Autodesk Inventor part; units mm, degrees
ref_plane "Work Plane1" through (30.1625, 0, 0) normal (0, 0, -1) x (1, 0, 0)
ref_plane "YZ Plane" through (0, 0, 0) normal (1, 0, 0) x (0, 1, 0)
ref_plane "XZ Plane" through (0, 0, 0) normal (0, 1, 0) x (-1, 0, 0)
sketch "Szkic1" plane through (0, 0, 0) normal (0, 0, 1) x (1, 0, 0)
  line L0 (-6, 0) -> (12, 0)
  line L1 (12, 0) -> (12, 5)
  line L2 (12, 5) -> (3, 5)
  line L3 (3, 5) -> (2.0797, 4.54)
  line L4 (2.0797, 4.54) -> (0, 4.54)
  line L5 (0, 4.54) -> (0, 8)
  line L6 (-9.6, 0) -> (15.6, 0)
  line L7 (0, -1.6) -> (0, 9.6)
  line L8 (-6, 0) -> (-6, 7.4751)
  line L9 (0, 8) -> (-6, 7.4751)
  line L10 (3, 5) -> (0, 5) construction
  dimension "d0" = 12
  dimension "d1" = 9
  dimension "d2" = 0.9203
  dimension "d3" = 6
  dimension "d4" = 10
  dimension "d5" = 9.08
  dimension "d9" = 16
  dimension "d10" = 5
revolve "Bryła" add sketch "Szkic1" angle 360 about axis through (-6, 0, 0) along (1, 0, 0)
sketch "Szkic2" plane through (-6, 0, 0) normal (-1, 0, 0) x (0, 0, 1)
  circle A0 centre (0, 0) radius 8
  line L0 (0, 0) -> (0, 7.4751)
  line L1 (-8, 1.25) -> (8, 1.25)
  line L2 (8, 1.25) -> (8, -1.25)
  line L3 (8, -1.25) -> (-8, -1.25)
  line L4 (-8, -1.25) -> (-8, 1.25)
  line L5 (-8, 0) -> (8, 0) construction
  line L6 (0, 1.25) -> (0, -1.25) construction
  dimension "d11" = 2.5
  dimension "d12" = 16
fillet "Zaokrąglenie1" radius 0.4 1 edges at (-6, -7.4751, 0)
extrude "Szczelina" cut sketch "Szkic2" against normal blind 2.4 contours A0 L3 L1 | L2 L3 A0 | A0 L1 L2 | A0 L4 L1 | L3 L4 A0
thread "Gwint"
chamfer "Faza1" distance 0.9202 distance2 0.9203 1 edges at (12, -5, 0) measured on face at (12, -0.8193, 1.889)
ref_plane "Work Plane1" through (30.1625, 0, 0) normal (0, 0, -1) x (1, 0, 0)
equation "\"d11\" = SBR"
equation "\"d12\" = KOD"
equation "\"d14\" = RR"
equation "\"d19\" = STI"
equation "\"d15\" = GEL"
equation "\"d17\" = -0.5 * SPD + 0.5 * GD"
equation "\"d0\" = NLG"
equation "\"d1\" = GEL"
equation "\"d3\" = KOH"
equation "\"d4\" = GD"
equation "\"d5\" = BDM"
equation "\"d9\" = KOD"
equation "\"d10\" = KEWI"
equation "\"GD\" = NND"
equation "\"NLG\" = 12"
equation "\"GEL\" = 9"
equation "\"KOD\" = 16"
equation "\"KOH\" = 6"
equation "\"GAL\" = 0.61345 * PTC"
equation "\"SPD\" = NND - 1.2269 * PTC"
equation "\"BDM\" = 9.08"
equation "\"GUL\" = 0.61345 * PTC"
equation "\"RR\" = 0.4"
equation "\"SBR\" = 2.5"
equation "\"STI\" = 2.4"
equation "\"KEWI\" = 5deg"
equation "\"PTC\" = 1.5"
equation "\"TOA\" = 30deg"
equation "\"GD1\" = THREADDIA - 1.2269 * PTC"
properties part number "ISO 1207 - M10 x 12" material "Stal nierdzewna 440C"
Read the model definition and answer for the solid it produces. Units are mm, in the model's axes. A direction names the side the tool comes from. Coordinates: 2 decimals unless noted, no trailing zeros. Loops run counter-clockwise (first coordinate to the right, second up) from the corner with the lowest first, then second, coordinate; pieces in that order, holes last. Notation, with made-up numbers: (32, -2.5) -> (41, -2.5) arc R38 cw to (41, 36.5) -> close; hole circle Ø2 at (-6, -18.75). An arc over 180 degrees is marked (long way). Write item = value, one per line. Start each with the question number.
1) The part is cut by section B-B, the plane y = 0. Determine the outline of the cut face in (x, z), plus the area to 3 significant figures.
2) Given P1, Ø3, axis at x = 7.5, z = -6, coming from the +Y side; P2, Ø1.9, axis at x = -5.5, z = 0, coming from the +Y side; P3, Ø3, axis at x = 8.5, z = -6, coming from the -Y side; P4, Ø6, axis at x = -1, z = 0.5, coming from the +Y side, each flat-ended and moving along its own axis, determine where each tip first touches the part or whether it passes through.
3) The part is cut by section A-A, the plane z = 0. Determine the outline of the cut face in (x, y).
4) Find the intervals of material crossed by L1, parallel to Y at x = -4.5, z = -0.5; L2, parallel to Y at x = 8.5, z = 0.25; L3, parallel to X at y = 0, z = -0.25, in increasing order. Write a range as from..to.
5) The mould has two halves that part along Y. Classify faces 4 (the face through (-3.4, -1.67, -7.52)), 5 (the face through (-5, -1.25, 0)), 6 (the face through (12, 0, 0)): pulls with the +Y half, pulls with the -Y half, needs draft (parallel to the pull), parting line crosses it, or undercut.
6) For faces 1 (the face through (1.025, -3.603, 2.763)), 2 (the face through (-3.6, 0, 0)), 3 (the face through (6.98, -1.08, 4.88)), determine the directions among +Z, -Z, +X, -X, +Y, -Y from which every point of the face is accessible in a straight line to the end or side of a thin tool.
7) The part is cut by section C-C, the plane x = 3.75. Determine the outline of the cut face in (y, z).
Result:
q1.outline = (-3.6, -7.69) -> (0, -8) -> (0, -4.54) -> (2.08, -4.54) -> (3, -5) -> (11.08, -5) -> (12, -4.08) -> (12, 4.08) -> (11.08, 5) -> (3, 5) -> (2.08, 4.54) -> (0, 4.54) -> (0, 8) -> (-3.6, 7.69) -> close
q1.area = 173 mm²
q2.P1 = 2.18
q2.P2 = 7.6
q2.P3 = -2.18
q2.P4 = 8
q3.outline = (-6, -7.11) arc R0.4 ccw to (-5.63, -7.51) -> (0, -8) -> (0, -4.54) -> (2.08, -4.54) -> (3, -5) -> (11.08, -5) -> (12, -4.08) -> (12, 4.08) -> (11.08, 5) -> (3, 5) -> (2.08, 4.54) -> (0, 4.54) -> (0, 8) -> (-5.63, 7.51) arc R0.4 ccw to (-6, 7.11) -> (-6, 1.25) -> (-3.6, 1.25) -> (-3.6, -1.25) -> (-6, -1.25) -> close
q4.L1 = -7.59..-1.25, 1.25..7.59
q4.L2 = -4.99..4.99
q4.L3 = -3.6..12
q5.face_4 = parting line crosses it
q5.face_5 = undercut
q5.face_6 = needs draft
q6.face_1 = none
q6.face_2 = +Z, -Z, -X
q6.face_3 = +X
q7.outline = circle Ø10 at (0, 0)
